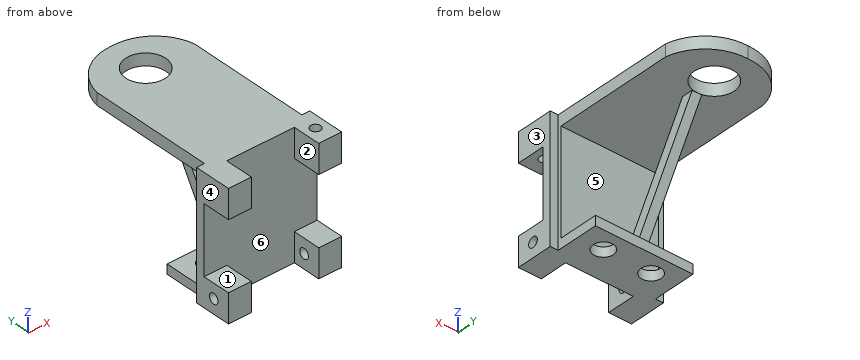
Autodesk Inventor part; units mm, degrees
ref_plane "Work Plane1" through (19.4945, 61.0616, 0) normal (1, 0, 0) x (0, 0, -1)
ref_plane "YZ Plane" through (0, 0, 0) normal (1, 0, 0) x (0, 1, 0)
ref_plane "XZ Plane" through (0, 0, 0) normal (0, 1, 0) x (-1, 0, 0)
sketch "Sketch1" plane through (0, 0, 0) normal (0, 0, 1) x (1, 0, 0)
  line L0 (0, 0) -> (38.989, 0)
  line L1 (0, 8.1026) -> (0, 61.0616)
  line L2 (38.989, 8.1026) -> (38.989, 61.0616)
  arc A0 (19.4945, 76.6064) -> (0, 61.0616) centre (18.7276, 57.5718) ccw
  arc A1 (38.989, 61.0616) -> (19.4945, 76.6064) centre (20.2614, 57.5718) ccw
  line L3 (0, 8.1026) -> (38.989, 8.1026)
  line L4 (0, 61.0616) -> (38.989, 61.0616)
  dimension "d3" = 19.05
  dimension "d4" = 19.05
extrude "Extrusion1" add sketch "Sketch1" against normal blind 4.8006
sketch "Sketch2" plane through (0, 0, 0) normal (0, 0, 1) x (1, 0, 0)
  line L0 (38.989, 8.1026) -> (0, 8.1026)
  line L1 (38.989, 61.0616) -> (38.989, 8.1026)
  line L2 (5.9944, 8.1026) -> (32.9946, 8.1026)
  line L3 (38.989, 11.5157) -> (38.989, 12.8778)
  line L4 (38.989, 12.8778) -> (0, 12.8778)
  line L5 (0, 12.8778) -> (0, 11.5157)
  line L6 (5.9944, 8.1026) -> (5.9944, 0)
  line L7 (5.9944, 0) -> (0, 0)
  line L8 (32.9946, 8.1026) -> (32.9946, 0)
  line L9 (32.9946, 0) -> (38.989, 0)
  line L10 (38.989, 0) -> (42.164, 0)
  line L11 (42.164, 0) -> (42.164, 11.5157)
  line L12 (42.164, 11.5157) -> (38.989, 11.5157)
  line L13 (38.989, 12.8778) -> (38.989, 11.5157)
  line L14 (0, 0) -> (-3.175, 0)
  line L15 (-3.175, 0) -> (-3.175, 11.5157)
  line L16 (-3.175, 11.5157) -> (0, 11.5157)
extrude "Extrusion2" add sketch "Sketch2" against normal blind 50.0126 contours L0 L6 L7 L14 L15 L16 L5 L4 L1
sketch "Sketch3" plane through (0, 0, -50.0126) normal (0, 0, -1) x (-1, 0, 0)
  line L0 (-38.989, 12.8778) -> (0, 12.8778)
  line L1 (-4.4958, 12.8778) -> (-34.4932, 12.8778)
  line L2 (-34.4932, 28.7528) -> (-4.4958, 28.7528)
  line L3 (-38.989, 8.1026) -> (-38.989, 61.0616)
  circle A0 centre (-28.9433, 20.8153) radius 4.0513
  circle A1 centre (-9.8425, 20.8153) radius 4.0513
  line L4 (-34.4932, 12.8778) -> (-38.989, 12.8778)
  line L5 (-38.989, 12.8778) -> (-38.989, 28.7528)
  line L6 (-38.989, 28.7528) -> (-34.4932, 28.7528)
  line L7 (-4.4958, 28.7528) -> (0, 28.7528)
  line L8 (0, 12.8778) -> (0, 61.0616)
  line L9 (0, 28.7528) -> (0, 12.8778)
  line L10 (0, 12.8778) -> (-4.4958, 12.8778)
  point P0 (0, 0)
  point P1 (-38.989, 0)
  dimension "d17" = 8.1026
  dimension "d19" = 8.1026
extrude "Extrusion3" add sketch "Sketch3" against normal blind 3.81
ref_plane "Work Plane1" through (19.4945, 61.0616, 0) normal (1, 0, 0) x (0, 0, -1)
sketch "Sketch6" plane through (0, 0, 0) normal (0, 0, 1) x (1, 0, 0)
  line L0 (0, 61.0616) -> (0, 0)
  arc A0 (38.989, 61.0616) -> (19.4945, 76.6064) centre (20.2614, 57.5718) ccw
  circle A1 centre (19.4945, 61.0616) radius 8
  dimension "d22" = 16
extrude "Extrusion4" cut sketch "Sketch6" against normal blind 5.3975
sketch "Sketch7" plane through (19.4945, 61.0616, 0) normal (1, 0, 0) x (0, 0, -1)
  line L0 (0, -8) -> (4.8006, -8)
  line L1 (4.8006, -8) -> (46.2026, -32.3088)
  line L2 (46.2026, -32.3088) -> (46.2026, -48.1838)
  line L3 (4.8006, 0) -> (4.8006, -48.1838)
  line L4 (46.2026, -44.2976) -> (46.2026, -36.195)
  line L5 (46.2026, -36.727) -> (4.8006, -12.4182)
  point P0 (0, -61.0616)
extrude "Extrusion5" add sketch "Sketch7" along normal mid plane 3.81
sketch "Sketch11" plane through (38.989, 61.0616, 0) normal (1, 0, 0) x (0, 0, -1)
  line L0 (0, -61.0616) -> (50.0126, -61.0616)
  line L1 (50.0126, -48.1838) -> (50.0126, -61.0616)
  circle A0 centre (25.0063, -57.2836) radius 2
  dimension "d54" = 4
extrude "Extrusion8" cut sketch "Sketch11" against normal blind 7.9375
extrude "Extrusion9" add sketch "Sketch2" against normal up to surface (50.0126 mm away) contours L1 L12 L11 L10 L9 L8 L0
sketch "Sketch12" plane through (42.164, 0, 0) normal (1, 0, 0) x (0, 0, -1)
  line L0 (0, 0) -> (50.0126, 0)
  line L1 (25.0063, 8.1026) -> (11.5062, 8.1026)
  line L2 (11.5062, 8.1026) -> (11.5062, 0)
  line L3 (25.0063, 8.1026) -> (38.5064, 8.1026)
  line L4 (0, 8.1026) -> (50.0126, 8.1026)
  line L5 (38.5064, 8.1026) -> (38.5064, 0)
  line L6 (11.5062, 0) -> (38.5064, 0)
  dimension "d63" = 13.5001
  dimension "d64" = 13.5001
extrude "Extrusion10" cut sketch "Sketch12" against normal up to surface (45.339 mm away)
sketch "Sketch13" plane through (0, 0, 0) normal (0, 0, 1) x (1, 0, 0)
  circle A0 centre (37.5793, 3.6) radius 2
  line L0 (32.9946, 0) -> (42.164, 0)
  line L1 (37.5793, 0) -> (37.5793, 1.6)
  line L2 (37.5793, 0) -> (39.1793, 0) construction
  point P0 (0, 0)
  dimension "d67" = 4
  dimension "d68" = 1.6
  dimension "d69" = 90
extrude "Extrusion11" cut sketch "Sketch13" against normal up to surface (11.5062 mm away)
sketch "Sketch14" plane through (42.164, 0, 0) normal (1, 0, 0) x (0, 0, -1)
  circle A0 centre (44.2595, 3.6) radius 2
  point P0 (0, 0)
  point P1 (38.5064, 0)
  point P2 (50.0126, 0)
  dimension "d73" = 4
extrude "Extrusion12" cut sketch "Sketch14" against normal up to surface (45.339 mm away)
sketch "Sketch15" plane through (0, 0, 0) normal (0, 0, 1) x (1, 0, 0)
  line L0 (-3.175, 0) -> (5.9944, 0)
  line L1 (-3.175, 0) -> (5.9944, 0)
  line L2 (5.9944, 0) -> (5.9944, -3.175)
  line L3 (5.9944, -3.175) -> (-3.175, -3.175)
  line L4 (-3.175, -3.175) -> (-3.175, 0)
  line L5 (32.9946, 0) -> (42.164, 0)
  line L6 (32.9946, 0) -> (42.164, 0)
  line L7 (42.164, 0) -> (42.164, -3.175)
  line L8 (42.164, -3.175) -> (32.9946, -3.175)
  line L9 (32.9946, -3.175) -> (32.9946, 0)
  point P0 (0, 0)
  dimension "d76" = 3.175
  dimension "d77" = 3.175
extrude "Extrusion13" add sketch "Sketch15" against normal up to surface (50.0126 mm away)
sketch "Sketch16" plane through (-3.175, 11.5157, -50.0126) normal (-1, 0, 0) x (0, 0, 1)
  line L0 (38.5064, -11.5157) -> (11.5062, -11.5157)
  line L1 (38.5064, -11.5157) -> (38.5064, -14.6907)
  line L2 (50.0126, -14.6907) -> (0, -14.6907)
  line L3 (11.5062, -11.5157) -> (38.5064, -11.5157)
  line L4 (38.5064, -11.5157) -> (38.5064, -14.6907)
  line L5 (38.5064, -14.6907) -> (11.5062, -14.6907)
  line L6 (11.5062, -14.6907) -> (11.5062, -11.5157)
  point P0 (50.0126, -11.5157)
extrude "Extrusion14" cut sketch "Sketch16" against normal up to surface (45.339 mm away)
properties part number "Transmitter + Reciever"
For this review, take the finished solid that the model builds, in its own axes (mm). Face numbers are marked on the shaded views. A direction names the side the tool comes from. Coordinates: 2 decimals unless noted, no trailing zeros. Write each loop counter-clockwise with the first axis right and the second up, starting at its lowest first coordinate (ties: lowest second). Pieces come first, ordered by that corner, then holes.
(1) Add section B-B on z = -7.5. Give the boundary of the cut face in (x, y) (1 decimal).
(2) Wall thickness on probe 1 along Z at (x, y) = (9, 27); probe 2 along X at (y, z) = (3.6, -5.5) (3 decimals); probe 3 along X at (y, z) = (1, -45.5) (3 decimals): over which ranges is each line inside the solid? List them lowest first.
(3) Add section A-A on y = 3.6. Give the boundary of the cut face in (x, z) (1 decimal).
(4) For pin 1 Ø4 at (x, z) = (6, -40.5) entering from +Y; pin 2 Ø2.5 at (x, z) = (40.5, -31) entering from +Y; pin 3 Ø8 at (y, z) = (12.5, -21) entering from -X (3 decimals); pin 4 Ø5 at (x, z) = (16, -20) entering from +Y, all flat-tipped, find the tip position at first contact; note any pin that passes through.
(5) Add section D-D on y = 31. Give the boundary of the cut face in (x, z), then the cut area to 3 significant figures.
(6) Tool access review of the marked faces 1, 2 and 3: name each direction out of +Z, -Z, +X, -X, +Y, -Y from which nothing blocks a thin tool from reaching the whole face with its end or side.
(7) The part is to be moulded in two halves that separate along X. For the marked faces 4, 5 and 6, say which applies: +X half, -X half, draft (parallel to the pull), parting line (faces both ways), or undercut.
(8) Add section C-C on y = 19.5. Give the boundary of the cut face in (x, z).
Answer sheet:
1. outline: (-3.2, -3.2) - (6, -3.2) - (6, 8.1) - (33, 8.1) - (33, -3.2) - (42.2, -3.2) - (42.2, 11.5) - (39, 11.5) - (39, 12.9) - (0, 12.9) - (0, 11.5) - (-3.2, 11.5) - close; (17.6, 47.1) - (21.4, 47.1) - (21.4, 51.5) - (17.6, 51.5) - close; hole circle Ø4 at (37.6, 3.6)
2. probe 1: z = -50.01 to -46.2, -4.8 to 0
2. probe 2: x = -3.175 to 5.994, 32.995 to 35.579, 39.579 to 42.164
2. probe 3: x = -3.175 to 5.994, 32.995 to 42.164
3. outline: (-3.2, -50) - (6, -50) - (6, -46.3) - (-3.2, -46.3) - close; (-3.2, -42.3) - (6, -42.3) - (6, -38.5) - (-3.2, -38.5) - close; (-3.2, -11.5) - (6, -11.5) - (6, 0) - (-3.2, 0) - close; (33, -50) - (42.2, -50) - (42.2, -46.3) - (33, -46.3) - close; (33, -42.3) - (42.2, -42.3) - (42.2, -38.5) - (33, -38.5) - close; (33, -11.5) - (35.6, -11.5) - (35.6, 0) - (33, 0) - close; (39.6, -11.5) - (42.2, -11.5) - (42.2, 0) - (39.6, 0) - close
4. pin 1: stops at y = 12.88
4. pin 2: stops at y = 11.52
4. pin 3: stops at x = -3.175
4. pin 4: stops at y = 45.27
5. outline: (0, -4.8) - (38.99, -4.8) - (38.99, 0) - (0, 0) - close; (17.59, -42.38) - (21.4, -42.38) - (21.4, -34.85) - (17.59, -34.85) - close
5. area: 216 mm2
6. face 1: +X, -X, -Y
6. face 2: +Z, -Z, -Y
6. face 3: +Z, -Z, +X, +Y, -Y
7. face 4: -X half
7. face 5: draft
7. face 6: undercut
8. outline: (0, -50.01) - (6.01, -50.01) - (6.01, -46.2) - (0, -46.2) - close; (0, -4.8) - (38.99, -4.8) - (38.99, 0) - (0, 0) - close; (13.67, -50.01) - (25.11, -50.01) - (25.11, -46.2) - (13.67, -46.2) - close; (32.78, -50.01) - (38.99, -50.01) - (38.99, -46.2) - (32.78, -46.2) - close
